Geometry: final body of the model. Coordinates: model frame, mm. A direction names the side the tool comes from. Round coordinates to 2 decimals unless told otherwise and drop trailing zeros. Write each loop counter-clockwise with the first axis right and the second up, starting at its lowest first coordinate (ties: lowest second). Pieces come first, ordered by that corner, then holes. Notation, with made-up numbers: (33, 39) - (77, 39) arc R32 ccw to (77, 69) - close; hole circle Ø11 at (29.25, 78). An arc over 180 degrees is marked (long way). Use a Markdown table: item, result. Add a question column.
Autodesk Inventor part; units mm, degrees
ref_plane "YZ Plane" through (0, 0, 0) normal (1, 0, 0) x (0, 1, 0)
ref_plane "XZ Plane" through (0, 0, 0) normal (0, 1, 0) x (-1, 0, 0)
ref_plane "XY Plane" through (0, 0, 0) normal (0, 0, 1) x (1, 0, 0)
sketch "Sketch1" plane through (0, 0, 0) normal (0, 0, 1) x (1, 0, 0)
  line L0 (-40.83, 19.81) -> (40.83, 19.81)
  line L1 (40.83, 19.81) -> (40.83, -19.81)
  line L2 (40.83, -19.81) -> (-40.83, -19.81)
  line L3 (-40.83, -19.81) -> (-40.83, 19.81)
  point P0 (0, 0)
  dimension "d0" = 81.66
  dimension "d1" = 39.62
  dimension "d2" = 19.81
  dimension "d3" = 40.83
extrude "Extrusion1" add sketch "Sketch1" along normal blind 1
sketch "Sketch2" plane through (0, 0, 1) normal (0, 0, 1) x (1, 0, 0)
  line L0 (-40.83, 19.81) -> (-40.83, -19.81)
  line L1 (-40.83, -19.81) -> (40.83, -19.81)
  point P0 (0, 0)
  point P1 (-15.83, 16.19)
  point P2 (4.17, -16.81)
  point P3 (29.17, -16.81)
  dimension "d6" = 25
  dimension "d7" = 36
  dimension "d8" = 45
  dimension "d9" = 3
  dimension "d10" = 3
  dimension "d11" = 70
hole "Hole1" at (-15.83, 16.19, 1) at (4.17, -16.81, 1) at (29.17, -16.81, 1) direction (0, 0, -1) diameter 2 depth 3 tip angle 118
sketch "Sketch3" plane through (0, 0, 1) normal (0, 0, 1) x (1, 0, 0)
  line L0 (-40.83, 19.81) -> (-40.83, -19.81)
  line L1 (-40.83, 13.19) -> (-12.83, 13.19)
  line L2 (-12.83, 13.19) -> (-12.83, -2.81)
  line L3 (-12.83, -2.81) -> (-40.83, -2.81)
  line L4 (-40.83, -2.81) -> (-40.83, 13.19)
  line L5 (-40.83, -19.81) -> (40.83, -19.81)
  line L6 (40.83, 19.81) -> (-40.83, 19.81)
  line L7 (-40.83, 19.81) -> (-20.83, 19.81)
  line L8 (-20.83, 19.81) -> (-20.83, 13.19)
  line L9 (-20.83, 13.19) -> (-40.83, 13.19)
  line L10 (-40.83, 13.19) -> (-40.83, 19.81)
  line L11 (-40.83, -19.81) -> (40.83, -19.81)
  line L12 (40.83, -19.81) -> (40.83, 19.81)
  line L13 (-20.83, 19.81) -> (40.83, 19.81)
  line L14 (40.83, 19.81) -> (40.83, -19.81)
  line L15 (40.83, -19.81) -> (-20.83, -19.81)
  line L16 (-20.83, -19.81) -> (-20.83, 19.81)
  line L17 (-40.83, -2.81) -> (-20.83, -2.81)
  line L18 (-20.83, -2.81) -> (-20.83, -19.81)
  line L19 (-20.83, -19.81) -> (-40.83, -19.81)
  line L20 (-40.83, -19.81) -> (-40.83, -2.81)
  point P0 (0, 0)
  point P1 (-0.83, -19.81)
  point P2 (-20.83, -2.81)
  dimension "d19" = 28
  dimension "d20" = 33
  dimension "d21" = 17
  dimension "d22" = 8
extrude "Extrusion2" cut sketch "Sketch3" against normal blind 1 contours L6 L8 L1 L0 | L1 L16 L3 L0 | L3 L16 L5 L0 | L1 L2 L3 L16
sketch "Sketch4" plane through (0, 0, 1) normal (0, 0, 1) x (1, 0, 0)
  line L0 (-12.83, -2.81) -> (-20.83, -2.81)
  line L1 (-20.83, -2.81) -> (-20.83, -19.81)
  line L2 (-15.83, -2.81) -> (-20.83, -2.81)
  line L3 (-20.83, -2.81) -> (-20.83, -19.81)
  line L4 (-20.83, -19.81) -> (-15.83, -19.81)
  line L5 (-15.83, -19.81) -> (-15.83, -2.81)
  line L6 (-12.83, 13.19) -> (-12.83, -2.81)
  point P0 (0, 0)
  dimension "d26" = 3
extrude "Extrusion3" cut sketch "Sketch4" against normal blind 1
sketch "Sketch5" plane through (0, 0, 1) normal (0, 0, 1) x (1, 0, 0)
  line L0 (-1.17, 16.81) -> (30.83, 16.81)
  line L1 (30.83, 16.81) -> (30.83, -5.81)
  line L2 (30.83, -5.81) -> (-1.17, -5.81)
  line L3 (-1.17, -5.81) -> (-1.17, 16.81)
  line L4 (40.83, -19.81) -> (40.83, 19.81)
  line L5 (40.83, 19.81) -> (-20.83, 19.81)
  line L6 (-15.83, -19.81) -> (40.83, -19.81)
  point P0 (0, 0)
  dimension "d29" = 10
  dimension "d30" = 42
  dimension "d31" = 3
  dimension "d32" = 14
extrude "Extrusion4" add sketch "Sketch5" along normal blind 3
sketch "Sketch6" plane through (0, 0, 4) normal (0, 0, 1) x (1, 0, 0)
  line L0 (0.83, 11.81) -> (28.83, 11.81)
  line L1 (28.83, 11.81) -> (28.83, -0.81)
  line L2 (28.83, -0.81) -> (0.83, -0.81)
  line L3 (0.83, -0.81) -> (0.83, 11.81)
  line L4 (-1.17, 16.81) -> (-1.17, -5.81)
  line L5 (30.83, -5.81) -> (30.83, 16.81)
  line L6 (30.83, 16.81) -> (-1.17, 16.81)
  line L7 (-1.17, -5.81) -> (30.83, -5.81)
  point P0 (0, 0)
  dimension "d35" = 2
  dimension "d36" = 2
  dimension "d37" = 5
  dimension "d38" = 5
extrude "Extrusion5" cut sketch "Sketch6" against normal blind 4 contours L0 L1 L2 L3
sketch "Sketch7" plane through (0, 0, 1) normal (0, 0, 1) x (1, 0, 0)
  line L0 (40.83, -19.81) -> (40.83, 19.81)
  line L1 (-10.17, -5.81) -> (40.83, -5.81)
  line L2 (40.83, -5.81) -> (40.83, -8.61)
  line L3 (40.83, -8.61) -> (-10.17, -8.61)
  line L4 (-10.17, -8.61) -> (-10.17, -5.81)
  line L5 (40.83, 19.81) -> (-20.83, 19.81)
  line L6 (-10.17, 19.81) -> (40.83, 19.81)
  line L7 (40.83, 19.81) -> (40.83, 16.81)
  line L8 (40.83, 16.81) -> (-10.17, 16.81)
  line L9 (-10.17, 16.81) -> (-10.17, 19.81)
  line L10 (30.83, 16.81) -> (-1.17, 16.81)
  line L11 (-1.17, -5.81) -> (30.83, -5.81)
  point P0 (0, 0)
  point P1 (40.83, -5.81)
  dimension "d41" = 3
  dimension "d42" = 51
  dimension "d43" = 2.8
extrude "Extrusion6" add sketch "Sketch7" along normal blind 5
sketch "Sketch8" plane through (40.83, -19.81, 0) normal (1, 0, 0) x (0, 0, -1)
  line L0 (0, 0) -> (0, 39.62)
  line L1 (0, 0) -> (-6, 0)
  line L2 (-6, 0) -> (-6, 39.62)
  line L3 (-6, 39.62) -> (0, 39.62)
  line L4 (0, 39.62) -> (0, 0)
  point P0 (0, 19.81)
extrude "Extrusion7" cut sketch "Sketch8" against normal blind 0.2
sketch "Sketch9" plane through (0, 0, 1) normal (0, 0, 1) x (1, 0, 0)
  line L0 (-10.17, 16.81) -> (40.63, 16.81)
  line L1 (-10.17, 16.81) -> (-1.17, 5.5) construction
  line L2 (-1.17, 16.81) -> (-1.17, -5.81)
  line L3 (-10.9525, 16.1873) -> (-1.9525, 4.8773)
  line L4 (-0.3875, 6.1227) -> (-9.3875, 17.4327)
  arc A0 (-9.3875, 17.4327) -> (-10.9525, 16.1873) centre (-10.17, 16.81) ccw
  arc A1 (-1.9525, 4.8773) -> (-0.3875, 6.1227) centre (-1.17, 5.5) ccw
  line L5 (-10.17, -5.81) -> (-1.17, -5.81)
  line L6 (-1.17, 5.5) -> (-10.17, -5.81) construction
  line L7 (-1.9525, 6.1227) -> (-10.9525, -5.1873)
  line L8 (-9.3875, -6.4327) -> (-0.3875, 4.8773)
  arc A2 (-0.3875, 4.8773) -> (-1.9525, 6.1227) centre (-1.17, 5.5) ccw
  arc A3 (-10.9525, -5.1873) -> (-9.3875, -6.4327) centre (-10.17, -5.81) ccw
  line L9 (-10.17, 19.81) -> (-10.17, 16.81)
  line L10 (-10.17, 19.81) -> (-10.17, -8.4856)
  point P0 (0, 0)
  point P1 (-5.67, 11.155)
  point P2 (-5.67, -0.155)
  point P3 (-10.17, 15.204)
  point P4 (-2.448, 5.5)
  point P5 (-10.17, -4.204)
  point P6 (-8.892, -5.81)
  point P7 (-1.17, 3.894)
  point P8 (-1.17, 7.106)
  point P9 (-8.892, 16.81)
  dimension "d48" = 2
  dimension "d49" = 2
extrude "Extrusion8" add sketch "Sketch9" along normal blind 2 contours L0 L4 L2 A2 L7 L3 L10 | L7 A2 L2 A1 L3 | L3 A1 L2 L8 L5 L10 L7
fillet "Fillet1" radius 1 6 edges at (-8.892, 16.81, 2) (-1.17, 7.106, 2) (-1.17, 16.81, 2.5) (-1.17, 3.894, 2) (-8.892, -5.81, 2) (-1.17, -5.81, 2.5)
fillet "Fillet2" radius 1 1 edges at (-2.448, 5.5, 2)
equation "\"BendRadius\" = Thickness"
equation "\"BendReliefWidth\" = Thickness"
equation "\"BendReliefDepth\" = 0.5 * Thickness"
equation "\"CornerReliefSize\" = 4 * Thickness"
equation "\"MinimumRemnant\" = 2 * Thickness"
equation "\"TransitionRadius\" = BendRadius"
equation "\"JacobiRadiusSize\" = BendRadius"
equation "\"GapSize\" = Thickness"
properties part number "gen2-hdmi-mount"
1) Section A-A, the plane y = -16.81. Return the cut outline in (x, z), then the cut area to 3 significant figures.
2) Material intervals for L1, parallel to X at y = -16.81, z = 0.7; L2, parallel to Y at x = 4.17, z = 0.6; L3, parallel to Y at x = 37, z = 2.1, sorted ascending. Write a range as from..to.
3) Draft query along Y for faces 1 (the cylindrical face through (28.494, -16.073, 0.493)), 2 (the flat face through (15, 18, 6)), 3 (the flat face through (16, 19.81, 3)). Return one class per face: released by +Y, released by -Y, zero draft, split by the parting line, or undercut.
4) Set-up query: faces 4 (the flat face through (0.83, 5, 2)), 5 (the cylindrical face through (-7.71, 16.26, 2.01)), 6 (the flat face through (16, -8.61, 3)), 7 (the flat face through (-6.61, 10.73, 1.99)), 8 (the flat face through (-10.17, -7, 3)). Return all of +Z, -Z, +X, -X, +Y, -Y with unobstructed straight access to the full face (end or side cutting, diameter ignored); none if empty.
5) Section B-B, the plane x = 11. Return the cut outline in (y, z).
6) Section C-C, the plane z = 4.8. Return the cut outline in (x, y).
7) Pin query (flat end, axial travel): P1, Ø3, axis at x = 37.5, y = 6.5, coming from the +Z side; P2, Ø1.8, axis at x = 4.17, y = -16.81, coming from the -Z side (3 decimals); P3, Ø0.8, axis at x = -18.5, z = 0.5, coming from the -Y side; P4, Ø1, axis at x = -9, z = 2, coming from the -Y side. Return the tip coordinate at first contact, or that it passes through.
8) Section D-D, the plane y = 3. Return the cut outline in (x, z).
Output values:
| question | item | result |
|---|---|---|
| 1 | outline | (-15.83, 0) - (3.17, 0) - (3.17, 1) - (-15.83, 1) - close; (5.17, 0) - (28.17, 0) - (28.17, 1) - (5.17, 1) - close; (30.17, 0) - (40.63, 0) - (40.63, 1) - (30.17, 1) - close |
| 1 | area | 52.5 mm^2 |
| 2 | L1 | x = -15.83..3.17, 5.17..28.17, 30.17..40.63 |
| 2 | L2 | y = -19.81..-17.81, -15.81..-0.81, 11.81..19.81 |
| 2 | L3 | y = -8.61..-5.81, 16.81..19.81 |
| 3 | face 1 | undercut |
| 3 | face 2 | zero draft |
| 3 | face 3 | released by +Y |
| 4 | face 4 | +Z, -Z |
| 4 | face 5 | +Z |
| 4 | face 6 | +Z, +X, -X, -Y |
| 4 | face 7 | +Z, -X |
| 4 | face 8 | +Z, -X, +Y, -Y |
| 5 | outline | (-19.81, 0) - (-0.81, 0) - (-0.81, 4) - (-5.81, 4) - (-5.81, 6) - (-8.61, 6) - (-8.61, 1) - (-19.81, 1) - close; (11.81, 0) - (19.81, 0) - (19.81, 6) - (16.81, 6) - (16.81, 4) - (11.81, 4) - close |
| 6 | outline | (-10.17, -8.61) - (40.63, -8.61) - (40.63, -5.81) - (-10.17, -5.81) - close; (-10.17, 16.81) - (40.63, 16.81) - (40.63, 19.81) - (-10.17, 19.81) - close |
| 7 | P1 | stops at z = 1 |
| 7 | P2 | passes through |
| 7 | P3 | stops at y = 13.19 |
| 7 | P4 | stops at y = -8.61 |
| 8 | outline | (-12.83, 0) - (0.83, 0) - (0.83, 4) - (-1.17, 4) - (-1.17, 3) - (-4.44, 3) - (-4.44, 1) - (-12.83, 1) - close; (28.83, 0) - (40.63, 0) - (40.63, 1) - (30.83, 1) - (30.83, 4) - (28.83, 4) - close |
